```python
from build123d import *

# Parameters (mm, degrees)
SKETCH_1_R      = 1.1
EXTRUDE_1_DEPTH = 2
FILLET_1_R      = 2


with BuildPart() as part:
    # 草圖1 → 填料-伸長1 (new body)
    with BuildSketch(Plane.XY):
        with BuildLine():
            Line((2.5, 15), (60, 8))
            ThreePointArc((60, 8), (68, 0), (60, -8))
            Line((60, -8), (2.5, -15))
            Line((2.5, -15), (-2.5, -15))
            Line((-2.5, -15), (-2.5, 15))
            Line((-2.5, 15), (2.5, 15))
        make_face()
        with Locations((0, 13)):
            Circle(SKETCH_1_R, mode=Mode.SUBTRACT)
        with Locations((0, -13)):
            Circle(SKETCH_1_R, mode=Mode.SUBTRACT)
        with Locations((12, 11)):
            Circle(SKETCH_1_R, mode=Mode.SUBTRACT)
        with Locations((24, 9)):
            Circle(SKETCH_1_R, mode=Mode.SUBTRACT)
        with Locations((36, 7)):
            Circle(SKETCH_1_R, mode=Mode.SUBTRACT)
        with Locations((48, 5)):
            Circle(SKETCH_1_R, mode=Mode.SUBTRACT)
        with Locations((60, 3)):
            Circle(SKETCH_1_R, mode=Mode.SUBTRACT)
        with Locations(Location((60, -3, 0), (0, 0, 180))):
            Circle(SKETCH_1_R, mode=Mode.SUBTRACT)
        with Locations(Location((48, -5, 0), (0, 0, 180))):
            Circle(SKETCH_1_R, mode=Mode.SUBTRACT)
        with Locations(Location((36, -7, 0), (0, 0, 180))):
            Circle(SKETCH_1_R, mode=Mode.SUBTRACT)
        with Locations(Location((24, -9, 0), (0, 0, 180))):
            Circle(SKETCH_1_R, mode=Mode.SUBTRACT)
        with Locations(Location((12, -11, 0), (0, 0, 180))):
            Circle(SKETCH_1_R, mode=Mode.SUBTRACT)
        Polygon((4.5, 0), (4.5, 7), (46.5, 1.5), (46.5, -1.5), (4.5, -7), align=None, mode=Mode.SUBTRACT)
    extrude(amount=EXTRUDE_1_DEPTH)

    # 圓角1
    # the kernel refuses this fillet: 2 mm, written as the material it adds along each edge
    with BuildSketch(Plane(origin=(46.5, -1.5, 0), x_dir=(0, 1, 0), z_dir=(0, 0, 1)), Plane(origin=(46.5, 1.5, 0), x_dir=(-0.9915344613221523, 0.12984379850647185, 0), z_dir=(0, 0, 1))) as fillet_1_piece_1:
        with BuildLine():
            CenterArc((FILLET_1_R * 0.877585434936, FILLET_1_R), FILLET_1_R, 187.460566126, 82.539433874)
            Line((-FILLET_1_R * 0.113949026386, FILLET_1_R * 0.870156201494), (0, 0))
            Line((0, 0), (FILLET_1_R * 0.877585434936, 0))
        make_face()
    extrude(amount=2)
    with BuildSketch(Plane(origin=(4.5, -7, 0), x_dir=(0, 1, 0), z_dir=(0, 0, 1))) as fillet_1_piece_2:
        with BuildLine():
            CenterArc((FILLET_1_R * 1.13949019684, -FILLET_1_R), FILLET_1_R, 90, 97.460566126)
            Line((FILLET_1_R * 0.147955735519, -FILLET_1_R * 1.12984379851), (0, 0))
            Line((0, 0), (FILLET_1_R * 1.13949019684, 0))
        make_face()
    extrude(amount=2)
    with BuildSketch(Plane(origin=(4.5, 7, 0), x_dir=(0, -1, 0), z_dir=(0, 0, 1))) as fillet_1_piece_3:
        with BuildLine():
            CenterArc((FILLET_1_R * 1.13949019684, FILLET_1_R), FILLET_1_R, 172.539433874, 97.460566126)
            Line((FILLET_1_R * 0.147955735519, FILLET_1_R * 1.12984379851), (0, 0))
            Line((0, 0), (FILLET_1_R * 1.13949019684, 0))
        make_face()
    extrude(amount=2)


solid = part.part
```
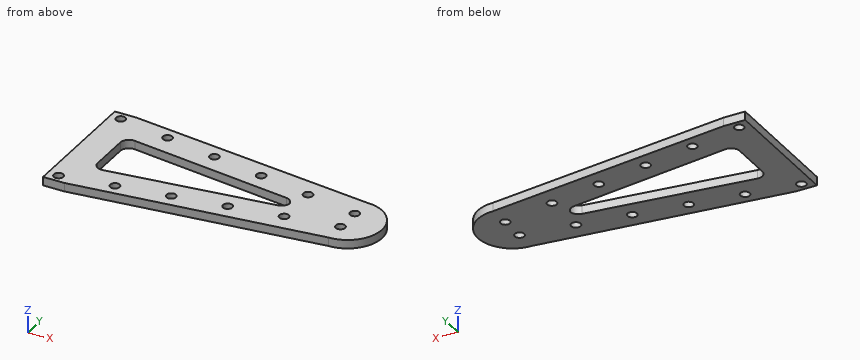
Verification items for the finished model (mm, model axes). Round coordinates to 2 decimals unless told otherwise and drop trailing zeros. Loops run counter-clockwise (first coordinate to the right, second up) from the corner with the lowest first, then second, coordinate; pieces in that order, holes last. Notation, with made-up numbers: (3, -9) -> (36, -9) arc R24 ccw to (36, 2) -> close; hole circle Ø2 at (59.25, -13). An arc over 180 degrees is marked (long way). Answer as a JSON object with one key per item and string values.
Q1. Scan lines: line 1 (Y direction, x = 12, z = 0.85); line 2 (Y direction, x = 59, z = 1.1); line 3 (Y direction, x = 48, z = 0.4). Record each from-to range of solid material in increasing order. Write a range as from..to.
Data:
{"line 1": "y = -13.84..-12.1, -9.9..-6.02, 6.02..9.9, 12.1..13.84", "line 2": "y = -8.12..-3.46, -2.54..2.54, 3.46..8.12", "line 3": "y = -9.46..-6.1, -3.9..3.9, 6.1..9.46"}
Q2. Section check B-B (y = -9). Record the boundary of the cut face in (x, z), then the cut area to 3 significant figures.
Data:
{"outline": "(-2.5, 0) -> (22.9, 0) -> (22.9, 2) -> (-2.5, 2) -> close; (25.1, 0) -> (51.79, 0) -> (51.79, 2) -> (25.1, 2) -> close", "area": "104 mm2"}
Q3. Section check D-D (x = 48). Record the boundary of the cut face in (y, z).
Data:
{"outline": "(-9.46, 0) -> (-6.1, 0) -> (-6.1, 2) -> (-9.46, 2) -> close; (-3.9, 0) -> (3.9, 0) -> (3.9, 2) -> (-3.9, 2) -> close; (6.1, 0) -> (9.46, 0) -> (9.46, 2) -> (6.1, 2) -> close"}
Q4. Section check C-C (x = 24). Record the boundary of the cut face in (y, z).
Data:
{"outline": "(-12.38, 0) -> (-10.1, 0) -> (-10.1, 2) -> (-12.38, 2) -> close; (-7.9, 0) -> (-4.45, 0) -> (-4.45, 2) -> (-7.9, 2) -> close; (4.45, 0) -> (7.9, 0) -> (7.9, 2) -> (4.45, 2) -> close; (10.1, 0) -> (12.38, 0) -> (12.38, 2) -> (10.1, 2) -> close"}
Q5. Section check A-A (x = 14). Record the boundary of the cut face in (y, z).
Data:
{"outline": "(-13.6, 0) -> (-5.76, 0) -> (-5.76, 2) -> (-13.6, 2) -> close; (5.76, 0) -> (13.6, 0) -> (13.6, 2) -> (5.76, 2) -> close"}
